Here's how the part is built. I have some questions about the finished solid (model axes, mm). A direction names the side the tool comes from. Coordinates: 2 decimals unless noted, no trailing zeros. Loops run counter-clockwise (first coordinate to the right, second up) from the corner with the lowest first, then second, coordinate; pieces in that order, holes last. Notation, with made-up numbers: (-4.75, 54.5) -> (27.25, 54.5) arc R32 cw to (27.25, 92.5) -> close; hole circle Ø9 at (14.5, -22.5). An arc over 180 degrees is marked (long way). Use CSV: the item, a comma, the result in double quotes. Start each with the question number.
Autodesk Inventor part; units mm, degrees
ref_plane "YZ Plane" through (0, 0, 0) normal (1, 0, 0) x (0, 1, 0)
ref_plane "XZ Plane" through (0, 0, 0) normal (0, 1, 0) x (-1, 0, 0)
ref_plane "XY Plane" through (0, 0, 0) normal (0, 0, 1) x (1, 0, 0)
sketch "Sketch1" plane through (0, 0, 0) normal (0, 1, 0) x (-1, 0, 0)
  circle A0 centre (0, 0) radius 41.5 construction
  line L0 (0, -41.5) -> (0, 41.5)
  arc A1 (0, 41.5) -> (0, -41.5) centre (0, 0) ccw
  circle A2 centre (-6, -34) radius 2.5
  circle A3 centre (-6, 34) radius 2.5
  line L1 (0, 0) -> (-41.5, 0) construction
  circle A4 centre (-35, 0) radius 2.5
  dimension "d0" = 83
  dimension "d1" = 83
  dimension "d2" = 5
  dimension "d3" = 6
  dimension "d4" = 34
  dimension "d5" = 34
  dimension "d6" = 35
extrude "Extrusion1" add sketch "Sketch1" along normal blind 2
sketch "Espacio9V" plane through (0, 2, 0) normal (0, 1, 0) x (1, 0, 0)
  line L0 (2.75, -24.25) -> (29.25, -24.25)
  line L1 (29.25, -24.25) -> (29.25, 24.25)
  line L2 (29.25, 24.25) -> (2.75, 24.25)
  line L3 (2.75, 24.25) -> (2.75, -24.25)
  line L4 (2.75, -24.25) -> (29.25, 24.25) construction
  line L5 (29.25, -24.25) -> (2.75, 24.25) construction
  line L6 (0, 0) -> (41.5, 0) construction
  arc A0 (0, -41.5) -> (0, 41.5) centre (0, 0) ccw construction
  point P0 (16, 0)
  dimension "d11" = 26.5
  dimension "d12" = 48.5
  dimension "d13" = 16
sketch "Sketch3" plane through (0, 0, 0) normal (0, 0, 1) x (1, 0, 0)
  line L0 (29.25, 2) -> (31.25, 2)
  line L1 (31.25, 2) -> (31.25, 6)
  line L2 (31.25, 6) -> (29.25, 6)
  line L3 (29.25, 6) -> (29.25, 2)
  line L4 (2.75, 2) -> (0.75, 2)
  line L5 (0.75, 2) -> (0.75, 6)
  line L6 (0.75, 6) -> (2.75, 6)
  line L7 (2.75, 6) -> (2.75, 2)
  point P0 (0, 0)
  point P1 (2.75, 2)
  dimension "d14" = 2
  dimension "d15" = 4
  dimension "d16" = 4
  dimension "d17" = 2
extrude "Extrusion2" add sketch "Sketch3" along normal mid plane 30
fillet "Fillet1" radius 1 8 edges at (30.25, 2, 15) (29.25, 2, 0) (30.25, 2, -15) (31.25, 2, 0) (2.75, 2, 0) (1.75, 2, 15) (1.75, 2, -15) (0.75, 2, 0)
fillet "Fillet2" radius 1 2 edges at (2.75, 6, 0) (29.25, 6, 0)
properties part number "_3DPrint"
1) I want a section at D-D, the plane x = 26. Please give me the cut outline in (y, z), plus the area to 3 significant figures.
2) For P1, Ø6.5, axis at x = 6, z = -34, coming from the +Y side; P2, Ø0.6, axis at y = 4.5, z = -7.5, coming from the -X side; P3, Ø1, axis at x = 30, y = 5, coming from the +Z side; P4, Ø3, axis at x = 7, y = 4.5, coming from the -Z side, each with a flat end and sliding along its axis, tell me the tip position at first contact or that it passes through.
3) I want a section at C-C, the plane z = 8.5. Please give me the cut outline in (x, y), plus the area to 3 significant figures.
4) Please list where these lines run through material, in increasing order: L1, parallel to Z at x = 6, y = 1.1; L2, parallel to Y at x = 7, z = 31; L3, parallel to X at y = 3.35, z = -9. Write a range as [from, to].
5) I want a section at B-B, the plane z = -34. Please give me the cut outline in (x, y), plus the area to 3 significant figures.
6) Which directions (+Z, -Z, +X, -X, +Y, -Y) give clear straight access to the entire face, cutting with the end or side of a thin tool? Please do faces 1 (the face through (31.25, 4, 0)), 2 (the face through (29.25, 4, 0)), 3 (the face through (2, 5, -15)).
7) I want a section at A-A, the plane y = 4.2. Please give me the cut outline in (x, z), plus the area to 3 significant figures.
8) Thinking about a two-plate mould opening in Z: for faces 4 (the face through (0.75, 4, 0)), 5 (the face through (30, 5, 15)), 6 (the face through (32.69, 0.99, 0.96)), which applies, pulls with the +Z half, pulls with the -Z half, needs draft (parallel to the pull), parting line crosses it, or undercut?
Return value:
1,outline,"(0, -32.35) -> (2, -32.35) -> (2, 32.35) -> (0, 32.35) -> close"
1,area,"129 mm²"
2,P1,"stops at y = 2"
2,P2,"stops at x = 0.75"
2,P3,"stops at z = 15"
2,P4,"passes through"
3,outline,"(0, 0) -> (40.62, 0) -> (40.62, 2) -> (32.25, 2) arc R1 cw to (31.25, 3) -> (31.25, 6) -> (30.25, 6) arc R1 ccw to (29.25, 5) -> (29.25, 3) arc R1 cw to (28.25, 2) -> (3.75, 2) arc R1 cw to (2.75, 3) -> (2.75, 5) arc R1 ccw to (1.75, 6) -> (0.75, 6) -> (0.75, 2.97) arc R1 cw to (0, 2) -> close"
3,area,"97.6 mm²"
4,L1,"z = [-41.06, -36.5], [-31.5, 31.5], [36.5, 41.06]"
4,L2,"y = [0, 2]"
4,L3,"x = [0.75, 2.75], [29.25, 31.25]"
5,outline,"(0, 0) -> (3.5, 0) -> (3.5, 2) -> (0, 2) -> close; (8.5, 0) -> (23.8, 0) -> (23.8, 2) -> (8.5, 2) -> close"
5,area,"37.6 mm²"
6,face 1,"+Z, -Z, +X, +Y"
6,face 2,"+Z, -Z, +Y"
6,face 3,"-Z, +X, -X, +Y"
7,outline,"(0.75, -15) -> (2.75, -15) -> (2.75, 15) -> (0.75, 15) -> close; (29.25, -15) -> (31.25, -15) -> (31.25, 15) -> (29.25, 15) -> close"
7,area,"120 mm²"
8,face 4,"needs draft"
8,face 5,"pulls with the +Z half"
8,face 6,"undercut"
